```python
from build123d import *

# Parameters (mm, degrees)
EXTRUDE_1_DEPTH             = 4
SKETCH_1_4_R                = 1.25
CUT_EXTRUDE_4_DEPTH         = 10
PATTERN_LINEAR_1_COUNT      = 2
PATTERN_LINEAR_1_PITCH      = 29
PATTERN_LINEAR_1_COUNT_DIR2 = 2
PATTERN_LINEAR_1_PITCH_DIR2 = 23
CUT_EXTRUDE_6_DEPTH         = 19
SKETCH_1_7_R                = 1.4
CUT_EXTRUDE_8_DEPTH         = 9
CUT_EXTRUDE_10_DEPTH        = 9
SKETCH_1_8_R                = 15
CUT_EXTRUDE_12_DEPTH        = 9


with BuildPart() as part:
    # Sketch 1 → Extrude 1 (new body)
    with BuildSketch(Plane.XY):
        with BuildLine():
            Line((160, -120), (-160, -120))
            ThreePointArc((-160, -120), (-167.071067812, -117.071067812), (-170, -110))
            Line((-170, -110), (-170, 110))
            ThreePointArc((-170, 110), (-167.071067812, 117.071067812), (-160, 120))
            Line((-160, 120), (160, 120))
            ThreePointArc((160, 120), (167.071067812, 117.071067812), (170, 110))
            Line((170, 110), (170, -110))
            ThreePointArc((170, -110), (167.071067812, -117.071067812), (160, -120))
        make_face()
    extrude(amount=EXTRUDE_1_DEPTH)

    # Sketch 1_4 → Cut-Extrude 4 (cut)
    with BuildSketch(Plane.XY):
        with Locations((-90.205317251, 11.5)):
            Circle(SKETCH_1_4_R)
    cut_extrude_4 = extrude(amount=CUT_EXTRUDE_4_DEPTH, mode=Mode.SUBTRACT)

    # Pattern Linear 1: Cut-Extrude 4 2 × 2
    with Locations(*[(i * PATTERN_LINEAR_1_PITCH, -j * PATTERN_LINEAR_1_PITCH_DIR2, 0) for i in range(PATTERN_LINEAR_1_COUNT) for j in range(PATTERN_LINEAR_1_COUNT_DIR2) if (i, j) != (0, 0)]):
        add(cut_extrude_4, mode=Mode.SUBTRACT)

    # Sketch 1_6 → Cut-Extrude 6 (cut)
    with BuildSketch(Plane.XY):
        with BuildLine():
            Line((151.8, -83), (151.8, 83))
            ThreePointArc((151.8, 83), (153.4, 84.600001349), (155, 83))
            Line((155, 83), (155, -83))
            ThreePointArc((155, -83), (153.4, -84.600001349), (151.8, -83))
        make_face()
    extrude(amount=CUT_EXTRUDE_6_DEPTH, mode=Mode.SUBTRACT)

    # Sketch 1_7 → Cut-Extrude 8 (cut)
    with BuildSketch(Plane.XY):
        with Locations((135, -95.25)):
            Circle(SKETCH_1_7_R)
        with Locations(Location((39.75, -95.25, 0), (0, 0, 180))):
            Circle(SKETCH_1_7_R)
        with Locations((135, 0)):
            Circle(SKETCH_1_7_R)
        with Locations(Location((39.75, 0, 0), (0, 0, 180))):
            Circle(SKETCH_1_7_R)
    extrude(amount=CUT_EXTRUDE_8_DEPTH, mode=Mode.SUBTRACT)

    # Sketch 3 → Cut-Extrude 10 (cut)
    with BuildSketch(Plane.XY):
        with BuildLine():
            Line((-34, -24), (-71, -24))
            ThreePointArc((-71, -24), (-72.6, -22.4), (-71, -20.8))
            Line((-71, -20.8), (-34, -20.8))
            ThreePointArc((-34, -20.8), (-32.4, -22.4), (-34, -24))
        make_face()
        with BuildLine():
            Line((-34, -94.570317046), (-71, -94.570317046))
            ThreePointArc((-71, -94.570317046), (-72.6, -96.170317046), (-71, -97.770317046))
            Line((-71, -97.770317046), (-34, -97.770317046))
            ThreePointArc((-34, -97.770317046), (-32.4, -96.170317046), (-34, -94.570317046))
        make_face()
    extrude(amount=CUT_EXTRUDE_10_DEPTH, mode=Mode.SUBTRACT)

    # Sketch 1_8 → Cut-Extrude 12 (cut)
    with BuildSketch(Plane.XY):
        Circle(SKETCH_1_8_R)
    extrude(amount=CUT_EXTRUDE_12_DEPTH, mode=Mode.SUBTRACT)


solid = part.part
```
Input: part model. Units: mm. Frame: model coordinates. Give positions to 0.01 mm unless a question says otherwise; leave off trailing zeros. Loops run counter-clockwise (first coordinate to the right, second up) from the corner with the lowest first, then second, coordinate; pieces in that order, holes last.
1) Contact query for a flat-ended pin moving along its axis: pin 1 (3 mm diameter, centred on x = -61.21, y = 11.5, fed in from -Z). Output: stop coordinate, or through.
A:
pin 1: stops at z = 0
2) Section query B-B on x = -1. Return the cut outline in (y, z).
A:
outline: (-120, 0) - (-14.97, 0) - (-14.97, 4) - (-120, 4) - close; (14.97, 0) - (120, 0) - (120, 4) - (14.97, 4) - close
3) Line query: L1, parallel to Y at x = 39.75, z = 2.75; L2, parallel to Y at x = -64.5, z = 3.35; L3, parallel to X at y = 54, z = 1.4. Output: solid intervals per line, ascending.
A:
L1: y = -120 to -96.65, -93.85 to -1.4, 1.4 to 120
L2: y = -120 to -97.77, -94.57 to -24, -20.8 to 120
L3: x = -170 to 151.8, 155 to 170
4) Section query A-A on z = 1.5. Count the separate pieces of the cut face and the enclosed holes in it, and give its area (3 significant figures).
A:
separate pieces: 1
enclosed holes: 12
area: 80,000 mm2
